Build history of the part. All positions in model axes, mm. Face numbers are marked on the shaded views. Round coordinates to 2 decimals unless told otherwise and drop trailing zeros. Order: outer loops, then holes, each group sorted by start corner. A loop starts at its lowest first (then second) coordinate and runs counter-clockwise, first axis right, second up. Notation, with made-up numbers: M 66,-26.5 L 78,-26.5 A16 ccw 78,-1.5 Z; hole C 24,17.25 d2. An arc over 180 degrees is marked long. Use CSV: the item, a comma, the result in double quotes.
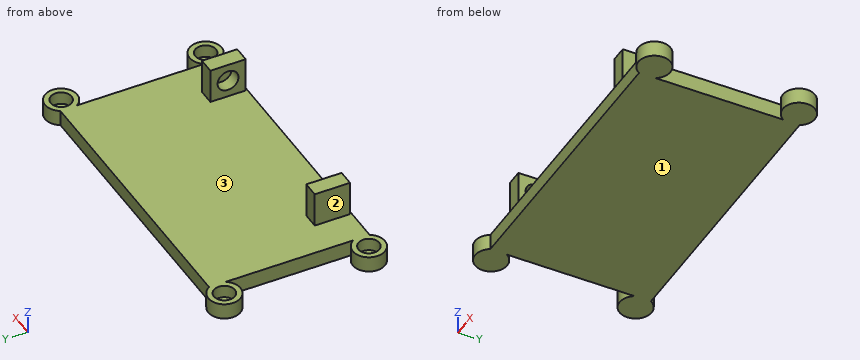
from build123d import *

# Parameters (mm, degrees)
CYLINDER093_R     = 10
CYLINDER093_DEPTH = 2
CYLINDER091_R     = 10
CYLINDER091_DEPTH = 2
CYLINDER090_R     = 10
CYLINDER090_DEPTH = 2
CYLINDER087_R     = 6.5
CYLINDER087_DEPTH = 10
CYLINDER086_R     = 10
CYLINDER086_DEPTH = 10
CYLINDER088_R     = 6.5
CYLINDER088_DEPTH = 10
CYLINDER089_R     = 10
CYLINDER089_DEPTH = 10
CYLINDER084_R     = 6.5
CYLINDER084_DEPTH = 10
CYLINDER082_R     = 10
CYLINDER082_DEPTH = 10
CYLINDER083_R     = 6.5
CYLINDER083_DEPTH = 10
CYLINDER085_R     = 10
CYLINDER085_DEPTH = 10
BOX025_W          = 177
BOX025_H          = 100
BOX025_DEPTH      = 10
CYLINDER069_R     = 2.6
CYLINDER069_DEPTH = 2
CYLINDER068_R     = 2.5
CYLINDER068_DEPTH = 5
CYLINDER071_R     = 2.6
CYLINDER071_DEPTH = 2
CYLINDER070_R     = 2.5
CYLINDER070_DEPTH = 5
CYLINDER073_R     = 2.6
CYLINDER073_DEPTH = 2
CYLINDER072_R     = 2.5
CYLINDER072_DEPTH = 5
CYLINDER066_R     = 2.6
CYLINDER066_DEPTH = 2
CYLINDER067_R     = 2.5
CYLINDER067_DEPTH = 5
CYLINDER063_R     = 6.5
CYLINDER063_DEPTH = 130
BOX024_W          = 10
BOX024_H          = 22
BOX024_DEPTH      = 22
BOX023_W          = 10
BOX023_H          = 22
BOX023_DEPTH      = 22
CYLINDER092_R     = 10
CYLINDER092_DEPTH = 2


with BuildPart() as cilindro093:
    # Cylinder093 → Cylinder093 (new body)
    with BuildSketch(Plane(origin=(97, 0, 0), x_dir=(1, 0, 0), z_dir=(0, 0, 1))):
        Circle(CYLINDER093_R)
    extrude(amount=CYLINDER093_DEPTH)


with BuildPart() as cilindro091:
    # Cylinder091 → Cylinder091 (new body)
    with BuildSketch(Plane(origin=(-97, 90, 0), x_dir=(1, 0, 0), z_dir=(0, 0, 1))):
        Circle(CYLINDER091_R)
    extrude(amount=CYLINDER091_DEPTH)


with BuildPart() as cilindro090:
    # Cylinder090 → Cylinder090 (new body)
    with BuildSketch(Plane(origin=(-97, 0, 0), x_dir=(1, 0, 0), z_dir=(0, 0, 1))):
        Circle(CYLINDER090_R)
    extrude(amount=CYLINDER090_DEPTH)


with BuildPart() as cilindro087:
    # Cylinder087 → Cylinder087 (new body)
    with BuildSketch(Plane(origin=(0, 20, 0), x_dir=(1, 0, 0), z_dir=(0, 0, 1))):
        Circle(CYLINDER087_R)
    extrude(amount=CYLINDER087_DEPTH)


with BuildPart() as obj1:
    # Cylinder086 → Cylinder086 (new body)
    with BuildSketch(Plane(origin=(0, 20, 0), x_dir=(1, 0, 0), z_dir=(0, 0, 1))):
        Circle(CYLINDER086_R)
    extrude(amount=CYLINDER086_DEPTH)

    # Cut051: cut Cilindro087
    add(cilindro087.part, mode=Mode.SUBTRACT)


with BuildPart() as obj1_1:
    # Cut051 placement: moved
    add(obj1.part.moved(Location((-97, -20, 0))))


with BuildPart() as cilindro088:
    # Cylinder088 → Cylinder088 (new body)
    with BuildSketch(Plane(origin=(0, 20, 0), x_dir=(1, 0, 0), z_dir=(0, 0, 1))):
        Circle(CYLINDER088_R)
    extrude(amount=CYLINDER088_DEPTH)


with BuildPart() as fusion034:
    # Cylinder089 → Cylinder089 (new body)
    with BuildSketch(Plane(origin=(0, 20, 0), x_dir=(1, 0, 0), z_dir=(0, 0, 1))):
        Circle(CYLINDER089_R)
    extrude(amount=CYLINDER089_DEPTH)

    # Cut052: cut Cilindro088
    add(cilindro088.part, mode=Mode.SUBTRACT)


with BuildPart() as fusion034_1:
    # Cut052 placement: moved
    add(fusion034.part.moved(Location((97, -20, 0))))

    # Fusion034: union obj1
    add(obj1_1.part)


with BuildPart() as fusion034_2:
    # Fusion034 placement: moved
    add(fusion034_1.part.moved(Location((0, 90, 0))))


with BuildPart() as cilindro084:
    # Cylinder084 → Cylinder084 (new body)
    with BuildSketch(Plane(origin=(0, 20, 0), x_dir=(1, 0, 0), z_dir=(0, 0, 1))):
        Circle(CYLINDER084_R)
    extrude(amount=CYLINDER084_DEPTH)


with BuildPart() as obj2:
    # Cylinder082 → Cylinder082 (new body)
    with BuildSketch(Plane(origin=(0, 20, 0), x_dir=(1, 0, 0), z_dir=(0, 0, 1))):
        Circle(CYLINDER082_R)
    extrude(amount=CYLINDER082_DEPTH)

    # Cut049: cut Cilindro084
    add(cilindro084.part, mode=Mode.SUBTRACT)


with BuildPart() as obj2_1:
    # Cut049 placement: moved
    add(obj2.part.moved(Location((-97, -20, 0))))


with BuildPart() as cilindro083:
    # Cylinder083 → Cylinder083 (new body)
    with BuildSketch(Plane(origin=(0, 20, 0), x_dir=(1, 0, 0), z_dir=(0, 0, 1))):
        Circle(CYLINDER083_R)
    extrude(amount=CYLINDER083_DEPTH)


with BuildPart() as fusion033:
    # Cylinder085 → Cylinder085 (new body)
    with BuildSketch(Plane(origin=(0, 20, 0), x_dir=(1, 0, 0), z_dir=(0, 0, 1))):
        Circle(CYLINDER085_R)
    extrude(amount=CYLINDER085_DEPTH)

    # Cut050: cut Cilindro083
    add(cilindro083.part, mode=Mode.SUBTRACT)


with BuildPart() as fusion033_1:
    # Cut050 placement: moved
    add(fusion033.part.moved(Location((97, -20, 0))))

    # Fusion033: union obj2
    add(obj2_1.part)


with BuildPart() as obj3:
    # Box025 → Box025 (new body)
    with BuildSketch(Plane(origin=(-88.5, -5, 0), x_dir=(1, 0, 0), z_dir=(0, 0, 1))):
        with Locations((88.5, 50)):
            Rectangle(BOX025_W, BOX025_H)
    extrude(amount=BOX025_DEPTH)


with BuildPart() as cilindro069:
    # Cylinder069 → Cylinder069 (new body)
    with BuildSketch(Plane.XY.offset(5)):
        Circle(CYLINDER069_R)
    extrude(amount=CYLINDER069_DEPTH)


with BuildPart() as obj4:
    # Cylinder068 → Cylinder068 (new body)
    with BuildSketch(Plane.XY):
        Circle(CYLINDER068_R)
    extrude(amount=CYLINDER068_DEPTH)

    # Fusion024: union Cilindro069
    add(cilindro069.part)


with BuildPart() as obj4_1:
    # Fusion024 placement: moved
    add(obj4.part.moved(Location((3, 8, -11))))


with BuildPart() as cilindro071:
    # Cylinder071 → Cylinder071 (new body)
    with BuildSketch(Plane.XY.offset(5)):
        Circle(CYLINDER071_R)
    extrude(amount=CYLINDER071_DEPTH)


with BuildPart() as obj5:
    # Cylinder070 → Cylinder070 (new body)
    with BuildSketch(Plane.XY):
        Circle(CYLINDER070_R)
    extrude(amount=CYLINDER070_DEPTH)

    # Fusion025: union Cilindro071
    add(cilindro071.part)


with BuildPart() as obj5_1:
    # Fusion025 placement: moved
    add(obj5.part.moved(Location((127, 8, -11))))


with BuildPart() as cilindro073:
    # Cylinder073 → Cylinder073 (new body)
    with BuildSketch(Plane.XY.offset(5)):
        Circle(CYLINDER073_R)
    extrude(amount=CYLINDER073_DEPTH)


with BuildPart() as obj6:
    # Cylinder072 → Cylinder072 (new body)
    with BuildSketch(Plane.XY):
        Circle(CYLINDER072_R)
    extrude(amount=CYLINDER072_DEPTH)

    # Fusion026: union Cilindro073
    add(cilindro073.part)


with BuildPart() as obj6_1:
    # Fusion026 placement: moved
    add(obj6.part.moved(Location((127, -8, -11))))


with BuildPart() as cilindro066:
    # Cylinder066 → Cylinder066 (new body)
    with BuildSketch(Plane.XY.offset(5)):
        Circle(CYLINDER066_R)
    extrude(amount=CYLINDER066_DEPTH)


with BuildPart() as fusion027:
    # Cylinder067 → Cylinder067 (new body)
    with BuildSketch(Plane.XY):
        Circle(CYLINDER067_R)
    extrude(amount=CYLINDER067_DEPTH)

    # Fusion023: union Cilindro066
    add(cilindro066.part)


with BuildPart() as fusion027_1:
    # Fusion023 placement: moved
    add(fusion027.part.moved(Location((3, -8, -11))))

    # Fusion027: union obj4, obj5, obj6
    add(obj4_1.part)
    add(obj5_1.part)
    add(obj6_1.part)


with BuildPart() as cilindro063:
    # Cylinder063 → Cylinder063 (new body)
    with BuildSketch(Plane(origin=(0, 0, 0), x_dir=(0, 0, -1), z_dir=(1, 0, 0))):
        Circle(CYLINDER063_R)
    extrude(amount=CYLINDER063_DEPTH)


with BuildPart() as cubo022:
    # Box024 → Box024 (new body)
    with BuildSketch(Plane(origin=(122, -11, -11), x_dir=(1, 0, 0), z_dir=(0, 0, 1))):
        with Locations((5, 11)):
            Rectangle(BOX024_W, BOX024_H)
    extrude(amount=BOX024_DEPTH)


with BuildPart() as obj7:
    # Box023 → Box023 (new body)
    with BuildSketch(Plane(origin=(-2, -11, -11), x_dir=(1, 0, 0), z_dir=(0, 0, 1))):
        with Locations((5, 11)):
            Rectangle(BOX023_W, BOX023_H)
    extrude(amount=BOX023_DEPTH)

    # Fusion021: union Cubo022
    add(cubo022.part)

    # Cut046: cut Cilindro063
    add(cilindro063.part, mode=Mode.SUBTRACT)

    # Cut047: cut Fusion027
    add(fusion027_1.part, mode=Mode.SUBTRACT)


with BuildPart() as obj7_1:
    # Cut047 placement: moved
    add(obj7.part.moved(Location((-65, 7, 21))))


with BuildPart() as obj8:
    # Cylinder092 → Cylinder092 (new body)
    with BuildSketch(Plane(origin=(97, 90, 0), x_dir=(1, 0, 0), z_dir=(0, 0, 1))):
        Circle(CYLINDER092_R)
    extrude(amount=CYLINDER092_DEPTH)

    # Fusion035: union Cilindro093, Cilindro091, Cilindro090, Fusion034, Fusion033, obj3, obj7
    add(cilindro093.part)
    add(cilindro091.part)
    add(cilindro090.part)
    add(fusion034_2.part)
    add(fusion033_1.part)
    add(obj3.part)
    add(obj7_1.part)


solid = obj8.part
(1) Cut at B-B, the plane x = 97. Give the cut face in (y, z).
Answer block:
outline,"M -10,0 L 10,0 L 10,10 L 6.5,10 L 6.5,2 L -6.5,2 L -6.5,10 L -10,10 Z; M 80,0 L 100,0 L 100,10 L 96.5,10 L 96.5,2 L 83.5,2 L 83.5,10 L 80,10 Z"
(2) Wall check: line 1 (Y direction, x = 62, z = 11.7); line 2 (Y direction, x = 97, z = 6); line 3 (X direction, y = 11, z = 19.5). Give the ranges that are in metal, low to high. Write a range as from..to.
Answer block:
line 1,"y = -4..-3.5, 1.5..12.5, 17.5..18"
line 2,"y = -10..-6.5, 6.5..10, 80..83.5, 96.5..100"
line 3,"x = -67..-65, 65..67"
(3) Drop flat-ended pins along their axis: pin 1 (8 mm diameter, centred on x = -9, z = 4, fed in from -Y); pin 2 (6 mm diameter, centred on x = -62, y = 15, fed in from -Z); pin 3 (17 mm diameter, centred on y = 7, z = 21, fed in from +X); pin 4 (10.5 mm diameter, centred on x = -98, y = -2, fed in from +Z). Give the stop position or say it passes through.
Answer block:
pin 1,"stops at y = -5"
pin 2,"stops at z = 0"
pin 3,"stops at x = 67"
pin 4,"stops at z = 10"
(4) Cut at C-C, the plane z = 21. Give the cut face in (x, y).
Answer block:
outline,"M -67,-4 L -57,-4 L -57,0.5 L -65,0.5 L -65,13.5 L -57,13.5 L -57,18 L -67,18 Z; M 57,-4 L 67,-4 L 67,18 L 57,18 L 57,13.5 L 65,13.5 L 65,0.5 L 57,0.5 Z"
(5) Cut at A-A, the plane z = 12.5. Give the cut face in (x, y).
Answer block:
outline,"M -67,-4 L -57,-4 L -57,18 L -67,18 Z; M 57,-4 L 67,-4 L 67,18 L 57,18 Z; hole C -62,-1 d5; hole C -62,15 d5; hole C 62,-1 d5; hole C 62,15 d5"
(6) Cut at D-D, the plane x = 62. Give the cut face in (y, z).
Answer block:
outline,"M -5,0 L 95,0 L 95,10 L 18,10 L 18,32 L -4,32 L -4,10 L -5,10 Z; hole M -3.6,15 L -3.5,15 L -3.5,10 L 1.5,10 L 1.5,15 L 1.6,15 L 1.6,17 L -3.6,17 Z; hole C 7,21 d13; hole M 12.4,15 L 12.5,15 L 12.5,10 L 17.5,10 L 17.5,15 L 17.6,15 L 17.6,17 L 12.4,17 Z"
(7) Two-plate mould, pull along X, no slides. Class the marked faces 1, 2 and 3: released by +X, released by -X, zero draft, split by the parting line, or undercut.
Answer block:
face 1,"zero draft"
face 2,"released by -X"
face 3,"undercut"
